Build history of the part. All positions in model axes, mm. A direction names the side the tool comes from. Coordinates: 2 decimals unless noted, no trailing zeros. Loops run counter-clockwise (first coordinate to the right, second up) from the corner with the lowest first, then second, coordinate; pieces in that order, holes last.
Item 1: Cut at A-A (z = 6.5). List the corners of the cut face in (x, y).
Item 2: Cut at C-C (x = 12.7). List the corners of the cut face in (y, z) (3 decimals).
Item 3: Cut at D-D (x = 131). List the corners of the cut face in (y, z) (3 decimals).
Item 4: Cut at B-B (y = 12.7). List the corners of the cut face in (x, z) (3 decimals).
Item 5: Flat gauge pins, fed straight in: pin 1 (8 mm diameter, centred on y = 12.7, z = 28.575, fed in from -X); pin 2 (1.5 mm diameter, centred on x = 77, y = 15, fed in from -Z) (3 decimals); pin 3 (1 mm diameter, centred on x = 24, y = 20, fed in from +Z) (3 decimals); pin 4 (4 mm diameter, centred on x = 99.5, z = -13, fed in from +Y). Where does each tip first touch, or does it go through?
Item 6: Drill centre lines: line 1 along Y through (x, z) = (38, 6); line 2 along Z through (x, y) = (107.5, 24) (3 decimals); line 3 along X through (y, z) = (4.5, 24). Where is each one in solid material? Low to high.
Item 7: 3-axis set-ups, long thin cutter, end or side, ignore diameter. For faces 1 (the face through (138, 13, -41.275)), 2 (the face through (61, 13, -10.795)), 3 (the face through (59, 13, 10.795)): which of +Z, -Z, +X, -X, +Y, -Y reach the whole face in a straight line?
Item 8: Mould opens along Y. For faces 4 (the face through (137.946, 12.848, 31.945)), 5 (the face through (148.59, 13, 1)), 6 (the face through (137.644, 1.811, -39.365)), 7 (the face through (137.946, 23.589, 39.365)) say: released by +Y, released by -Y, zero draft, split by the parting line, or undercut.
from build123d import *

# Parameters (mm, degrees)
BOSS_EXTRUDE1_DEPTH = 25.4
FILLET1_R           = 6.35
SKETCH2_R           = 3.3734375
CUT_EXTRUDE1_DEPTH  = 160.484898972
SKETCH3_R           = 3.3734375
CUT_EXTRUDE2_DEPTH  = 157.293869761
FILLET2_R           = 6.35
FILLET3_R           = 2.54


with BuildPart() as part:
    # Sketch1 → Boss-Extrude1 (new body)
    with BuildSketch(Plane(origin=(0, 0, 0), x_dir=(1, 0, 0), z_dir=(0, 1, 0))):
        Polygon((0, 10.795), (0, -10.795), (127, -10.795), (127, -41.275), (148.59, -41.275), (148.59, 41.275), (127, 41.275), (127, 10.795), align=None)
    extrude(amount=BOSS_EXTRUDE1_DEPTH)

    # Fillet1
    fillet1_edges = [part.edges().sort_by_distance(p)[0] for p in [
        (127, 12.7, -10.795),
        (127, 12.7, 10.795),
    ]]
    fillet(fillet1_edges, radius=FILLET1_R)

    # Sketch2 → Cut-Extrude1 (cut, through all)
    with BuildSketch(Plane.XY.offset(10.795)):
        with Locations((12.7, 12.7)):
            Circle(SKETCH2_R)
        with Locations((38.1, 12.7)):
            Circle(SKETCH2_R)
    extrude(amount=-CUT_EXTRUDE1_DEPTH, mode=Mode.SUBTRACT)

    # Sketch3 → Cut-Extrude2 (cut, through all)
    with BuildSketch(Plane(origin=(148.59, 0, 0), x_dir=(0, 0, -1), z_dir=(1, 0, 0))):
        with Locations((-28.575, 12.7)):
            Circle(SKETCH3_R)
        with Locations((28.575, 12.7)):
            Circle(SKETCH3_R)
    extrude(amount=-CUT_EXTRUDE2_DEPTH, mode=Mode.SUBTRACT)

    # Fillet2
    fillet2_edges = [part.edges().sort_by_distance(p)[0] for p in [
        (137.795, 25.4, 41.275),
        (137.795, 25.4, -41.275),
        (137.795, 0, -41.275),
        (137.795, 0, 41.275),
    ]]
    fillet(fillet2_edges, radius=FILLET2_R)

    # Fillet3
    fillet3_edges = [part.edges().sort_by_distance(p)[0] for p in [
        (0, 0, 0),
        (0, 25.4, 0),
    ]]
    fillet(fillet3_edges, radius=FILLET3_R)


solid = part.part
Filled sheet:
1. outline: (0, 2.54) arc R2.54 ccw to (2.54, 0) - (148.59, 0) - (148.59, 25.4) - (2.54, 25.4) arc R2.54 ccw to (0, 22.86) - close; hole circle Ø6.75 at (12.7, 12.7); hole circle Ø6.75 at (38.1, 12.7)
2. outline: (0, -10.795) - (9.327, -10.795) - (9.327, 10.795) - (0, 10.795) - close; (16.073, -10.795) - (25.4, -10.795) - (25.4, 10.795) - (16.073, 10.795) - close
3. outline: (0, -34.925) arc R6.35 ccw to (6.35, -41.275) - (19.05, -41.275) arc R6.35 ccw to (25.4, -34.925) - (25.4, 34.925) arc R6.35 ccw to (19.05, 41.275) - (6.35, 41.275) arc R6.35 ccw to (0, 34.925) - close; hole circle Ø6.747 at (12.7, -28.575); hole circle Ø6.747 at (12.7, 28.575)
4. outline: (0, -10.795) - (9.327, -10.795) - (9.327, 10.795) - (0, 10.795) - close; (16.073, -10.795) - (34.727, -10.795) - (34.727, 10.795) - (16.073, 10.795) - close; (41.473, -10.795) - (120.65, -10.795) arc R6.35 cw to (127, -17.145) - (127, -25.202) - (148.59, -25.202) - (148.59, 25.202) - (127, 25.202) - (127, 17.145) arc R6.35 cw to (120.65, 10.795) - (41.473, 10.795) - close; (127, -41.275) - (148.59, -41.275) - (148.59, -31.948) - (127, -31.948) - close; (127, 31.948) - (148.59, 31.948) - (148.59, 41.275) - (127, 41.275) - close
5. pin 1: stops at x = 127
5. pin 2: stops at z = -10.795
5. pin 3: stops at z = 10.795
5. pin 4: passes through
6. line 1: y = 0 to 9.33, 16.07 to 25.4
6. line 2: z = -10.795 to 10.795
6. line 3: x = 127 to 148.59
7. face 1: -Z, +X, -X, +Y, -Y
7. face 2: -Z, -X, +Y, -Y
7. face 3: +Z, -X, +Y, -Y
8. face 4: undercut
8. face 5: zero draft
8. face 6: released by -Y
8. face 7: released by +Y
